Autodesk Inventor part; units mm, degrees
ref_plane "YZ Plane" through (0, 0, 0) normal (1, 0, 0) x (0, 1, 0)
ref_plane "XZ Plane" through (0, 0, 0) normal (0, 1, 0) x (-1, 0, 0)
ref_plane "XY Plane" through (0, 0, 0) normal (0, 0, 1) x (1, 0, 0)
sketch "Náčrt1" plane through (0, 0, 0) normal (1, 0, 0) x (0, 1, 0)
  line L0 (1.5, 15) -> (-1.5, 15)
  line L1 (-1.5, 15) -> (-1.5, -15)
  line L2 (-1.5, -15) -> (1.5, -15)
  line L3 (1.5, -15) -> (1.5, 15)
  line L4 (1.5, 15) -> (-1.5, -15) construction
  line L5 (-1.5, 15) -> (1.5, -15) construction
  line L6 (-1.5, 15) -> (1.5, 8.5665)
  point P0 (0, 0)
  dimension "d0" = 3
  dimension "d1" = 30
  dimension "d2" = 25
extrude "Vysunutí1" add sketch "Náčrt1" along normal mid plane 99 contours L6 L3 L2 L1
sketch "Náčrt2" plane through (-49.5, -1.5, -15) normal (0, -1, 0) x (1, 0, 0)
  circle A0 centre (84.5, 7) radius 1.5
  circle A1 centre (49.5, 7) radius 1.5
  circle A2 centre (14.5, 7) radius 1.5
  line L0 (0, 0) -> (99, 0)
  line L1 (99, 30) -> (99, 0)
  line L2 (0, 30) -> (99, 30)
  line L3 (0, 0) -> (0, 30)
  line L4 (99, 7) -> (0, 7) construction
  line L5 (49.5, 0) -> (49.5, 30) construction
  point P0 (49.5, 15)
  dimension "d5" = 7
  dimension "d6" = 3
  dimension "d7" = 35
  dimension "d8" = 3
extrude "Vysunutí2" cut sketch "Náčrt2" against normal through all contours A0 | A1 | A2
thread "Závit1"
thread "Závit2"
thread "Závit3"
chamfer "Zkosení1" distance 0.5 angle 45 3 edges at (-36.5, 1.5, -8) (-1.5, 1.5, -8) (33.5, 1.5, -8)
sketch "Náčrt3" plane through (-49.5, -1.5, -15) normal (0, -1, 0) x (1, 0, 0)
  circle A0 centre (14.5, 7) radius 1.5
  circle A1 centre (49.5, 7) radius 1.5
  circle A2 centre (84.5, 7) radius 1.5
  line L0 (0, 0) -> (99, 0)
  line L1 (99, 30) -> (99, 0)
  line L2 (0, 30) -> (99, 30)
  line L3 (0, 0) -> (0, 30)
  line L4 (98.5, 0.5) -> (53.2335, 0.5) construction
  line L5 (53.2335, 0.5) -> (53.2335, 9.4631) construction
  line L6 (53.2335, 9.4631) -> (98.5, 9.4631) construction
  line L7 (98.5, 9.4631) -> (98.5, 0.5) construction
  point P0 (49.5, 15)
  dimension "d0" = 3
  dimension "d1" = 30
  dimension "d2" = 25
  dimension "d22" = 0.5
  dimension "d23" = 0.5
properties part number "Knife" material "Ocel, uhlík"
Can you work these out from the model? Positions are in its coordinate system, mm. Coordinates: 2 decimals unless noted, no trailing zeros. Order: outer loops, then holes, each group sorted by start corner. A loop starts at its lowest first (then second) coordinate and runs counter-clockwise, first axis right, second up.
1. If we section it at A-A (x = -35): Please give me the cut outline in (y, z), then the cut area to 3 significant figures.
2. I need wall thicknesses on line 1 (Z direction, x = -35, y = 0.15); line 2 (Z direction, x = 35, y = -1.2); line 3 (Z direction, x = -3, y = 1.2). Which ranges of each line are inside material? Lowest first, please.
3. If we section it at D-D (x = -23.5): Please give me the cut outline in (y, z).
4. Thinking about a two-plate mould opening in Z: for faces 1 (the face through (-0.325, -0.268, -9.464)), 2 (the face through (-1, 0, -15)), 3 (the face through (-49.5, 0, 0)), which applies, +Z half, -Z half, draft (parallel to the pull), parting line (faces both ways), or undercut?
5. If we section it at B-B (z = -8): Please give me the cut outline in (x, y).
6. If we section it at C-C (y = -0.75): Please give me the cut outline in (x, z).
Entries:
1. outline: (-1.5, -15) - (1.5, -15) - (1.5, -10) - (1, -9.5) - (-1.5, -9.5) - close; (-1.5, -6.5) - (1, -6.5) - (1.5, -6) - (1.5, 8.57) - (-1.5, 15) - close
1. area: 71.1 mm2
2. line 1: z = -15 to -9.5, -6.5 to 11.46
2. line 2: z = -15 to -9.5, -6.5 to 14.36
2. line 3: z = -15 to 9.21
3. outline: (-1.5, -15) - (1.5, -15) - (1.5, 8.57) - (-1.5, 15) - close
4. face 1: undercut
4. face 2: -Z half
4. face 3: draft
5. outline: (-49.5, -1.5) - (-36.5, -1.5) - (-36.5, 1) - (-37, 1.5) - (-49.5, 1.5) - close; (-33.5, -1.5) - (-1.5, -1.5) - (-1.5, 1) - (-2, 1.5) - (-33, 1.5) - (-33.5, 1) - close; (1.5, -1.5) - (33.5, -1.5) - (33.5, 1) - (33, 1.5) - (2, 1.5) - (1.5, 1) - close; (36.5, -1.5) - (49.5, -1.5) - (49.5, 1.5) - (37, 1.5) - (36.5, 1) - close
6. outline: (-49.5, -15) - (49.5, -15) - (49.5, 13.39) - (-49.5, 13.39) - close; hole circle Ø3 at (-35, -8); hole circle Ø3 at (0, -8); hole circle Ø3 at (35, -8)
